```python
from build123d import *

# Parameters (mm, degrees)
SKETCH1_R           = 3
BOSS_EXTRUDE1_DEPTH = 4


with BuildPart() as part:
    # Sketch1 → Boss-Extrude1 (new body)
    with BuildSketch(Plane.XY):
        with BuildLine():
            Line((-14.162950904, 14.142135624), (-14.121320344, 14.183766184))
            ThreePointArc((-14.121320344, 14.183766184), (-10.851949703, 14.834084438), (-9, 12.062445841))
            Line((-9, 12.062445841), (-9, -12.062445841))
            ThreePointArc((-9, -12.062445841), (-10.851949703, -14.834084438), (-14.121320344, -14.183766184))
            Line((-14.121320344, -14.183766184), (-14.162950904, -14.142135624))
            Line((-14.162950904, -14.142135624), (-28.305086528, -28.284271247))
            Line((-28.305086528, -28.284271247), (-0.02081528, -56.568542495))
            Line((-0.02081528, -56.568542495), (14.121320344, -42.426406871))
            Line((14.121320344, -42.426406871), (9.878679656, -38.183766184))
            ThreePointArc((9.878679656, -38.183766184), (9.228361402, -37.210496138), (9, -36.062445841))
            Line((9, -36.062445841), (9, 36.062445841))
            ThreePointArc((9, 36.062445841), (9.228361402, 37.210496138), (9.878679656, 38.183766184))
            Line((9.878679656, 38.183766184), (14.121320344, 42.426406871))
            Line((14.121320344, 42.426406871), (-0.02081528, 56.568542495))
            Line((-0.02081528, 56.568542495), (-28.305086528, 28.284271247))
            Line((-28.305086528, 28.284271247), (-14.162950904, 14.142135624))
        make_face()
        with Locations((-0.02081528, 42.426406871)):
            Circle(SKETCH1_R, mode=Mode.SUBTRACT)
        with Locations((-14.162950904, 28.284271247)):
            Circle(SKETCH1_R, mode=Mode.SUBTRACT)
        with Locations((-14.162950904, -28.284271247)):
            Circle(SKETCH1_R, mode=Mode.SUBTRACT)
        with Locations((-0.02081528, -42.426406871)):
            Circle(SKETCH1_R, mode=Mode.SUBTRACT)
    extrude(amount=BOSS_EXTRUDE1_DEPTH)


solid = part.part
```
The model under review builds one solid part; all positions refer to its coordinate system, in mm. A direction names the side the tool comes from. Give positions to 0.01 mm unless a question says otherwise; leave off trailing zeros. Write each loop counter-clockwise with the first axis right and the second up, starting at its lowest first coordinate (ties: lowest second). Pieces come first, ordered by that corner, then holes. Notation, with made-up numbers: M 84.25,44 L 106.25,44 A32 cw 106.25,75 Z; hole C 81,-26.75 d8. An arc over 180 degrees is marked long. Write item = value, one per line. Start each with the question number.
Q1. Machinability: for faces 4 (the face through (11.97, 40.275, 1.972)), 5 (the face through (-14.36, -42.23, 1.97)), 6 (the face through (-10.898, 14.853, 1.972)), 7 (the face through (7.15, 49.4, 1.97)), 8 (the face through (-21.33, 21.31, 1.97)), which of the approach directions +Z, -Z, +X, -X, +Y, -Y give a long, thin tool a straight path to every point of the face, cutting with its end or side? Answer none if there is none.
Q2. We need section D-D (x = -1.5). State the section outline as (y, z) points.
Q3. We need section B-B (y = -40.5). State the section outline as (x, z) points, plus the area to 3 significant figures.
Q4. We need section A-A (z = 2.4). State the section outline as (x, y) points.
Q5. Clearance check with a flat-ended pin moving along its axis: pin 1 (5 mm diameter, centred on x = -0.02, y = 42.43, fed in from +Z). State where the tip first meets the part, or that it passes through.
Q6. We need section C-C (x = -10). State the section outline as (y, z) points.
Q7. Mouldability with a two-part tool opening along X and no side actions: class faces 1 (the face through (-3, 1, 0)), 2 (the face through (-13.965, 42.624, 1.972)), 3 (the face through (-2.232, -40.399, 1.972)) as released by +X, released by -X, zero draft, split by the parting line, or undercut.
Q8. For line 1 (Y direction, x = -16.5, z = 3.1); line 2 (Y direction, x = -14.5, z = 1.7); line 3 (Y direction, x = 2.5, z = 1.2), list the stretches that pass through material, from the lowest coordinate up.
Result set:
q1.face_4 = +Z, -Z, +X
q1.face_5 = +Z, -Z, -X, -Y
q1.face_6 = +Z, -Z
q1.face_7 = +Z, -Z, +X, +Y
q1.face_8 = +Z, -Z, -X
q2.outline = M -55.09,0 L -45.04,0 L -45.04,4 L -55.09,4 Z; M -39.82,0 L 39.82,0 L 39.82,4 L -39.82,4 Z; M 45.04,0 L 55.09,0 L 55.09,4 L 45.04,4 Z
q3.outline = M -16.09,0 L -2.32,0 L -2.32,4 L -16.09,4 Z; M 2.28,0 L 12.19,0 L 12.19,4 L 2.28,4 Z
q3.area = 94.7 mm2
q4.outline = M -28.31,-28.28 L -0.02,-56.57 L 14.12,-42.43 L 9.88,-38.18 A3 cw 9,-36.06 L 9,36.06 A3 cw 9.88,38.18 L 14.12,42.43 L -0.02,56.57 L -28.31,28.28 L -14.16,14.14 L -14.12,14.18 A3 cw -9,12.06 L -9,-12.06 A3 cw -14.12,-14.18 L -14.16,-14.14 Z; hole C -14.16,-28.28 d6; hole C -14.16,28.28 d6; hole C -0.02,-42.43 d6; hole C -0.02,42.43 d6
q5.pin_1 = through
q6.outline = M -46.59,0 L -14.3,0 L -14.3,4 L -46.59,4 Z; M 14.3,0 L 46.59,0 L 46.59,4 L 14.3,4 Z
q7.face_1 = zero draft
q7.face_2 = released by -X
q7.face_3 = undercut
q8.line_1 = -40.09 to -30.17, -26.4 to -16.48, 16.48 to 26.4, 30.17 to 40.09
q8.line_2 = -42.09 to -31.27, -25.3 to -14.48, 14.48 to 25.3, 31.27 to 42.09
q8.line_3 = -54.05 to -44.05, -40.8 to 40.8, 44.05 to 54.05
